Check sheet for the drawn part. Datum: minimum x, y, z corner. Units: mm. A direction names the side the tool comes from. Round coordinates to 2 decimals unless told otherwise and drop trailing zeros. Write each loop counter-clockwise with the first axis right and the second up, starting at its lowest first coordinate (ties: lowest second). Pieces come first, ordered by that corner, then holes.
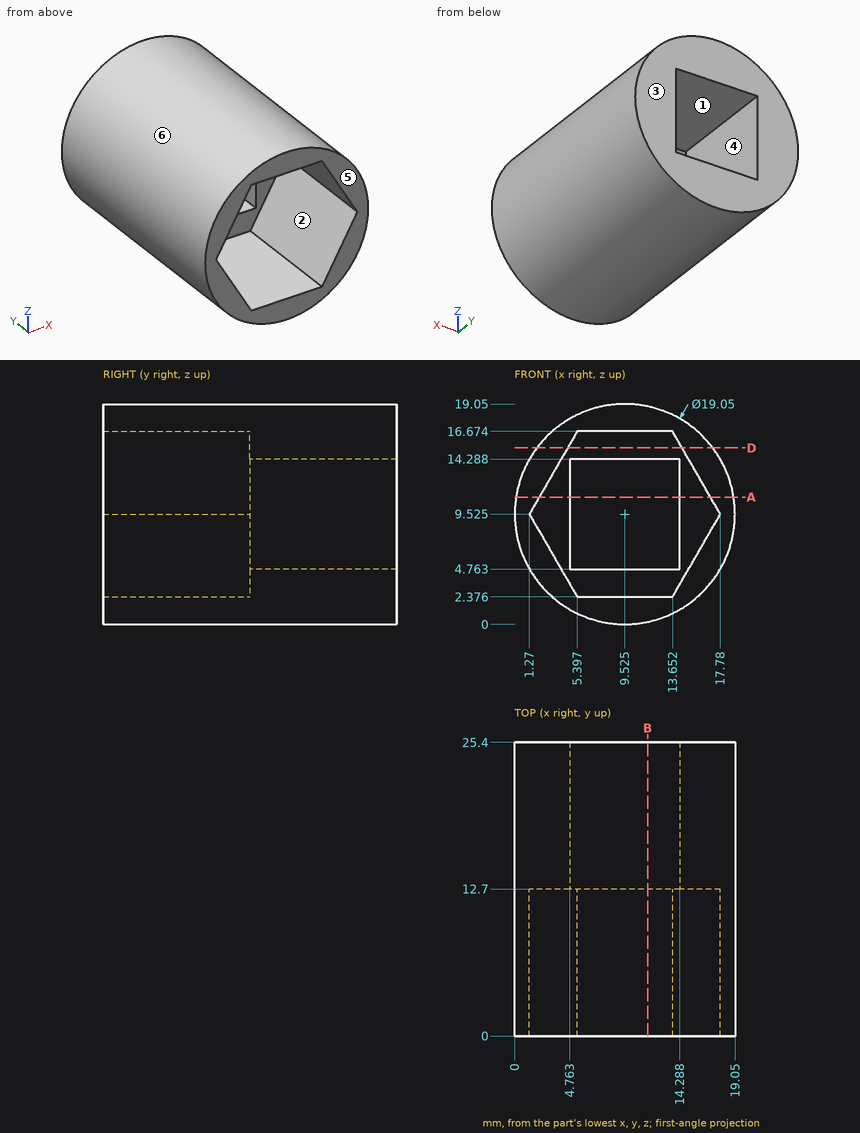
1. Sectioned sample at B-B, the plane x = 11.5. Enter the section's corners in (y, z) (1 decimal), plus the area to 3 significant figures.
2. Sectioned sample at D-D, the plane z = 15.25. Enter the section's corners in (x, y) (1 decimal).
3. Release check for a two-part mould opening along Z. For the marked faces 4, 5 and 6 record: released by +Z, released by -Z, zero draft, split by the parting line, or undercut.
4. Scan lines: line 1 along X through (y, z) = (16.75, 11) (1 decimal); line 2 along X through (y, z) = (1.5, 5) (1 decimal); line 3 along Z through (x, y) = (6, 13) (1 decimal). Record each from-to range of solid material in increasing order.
5. Sectioned sample at A-A, the plane z = 11. Enter the section's corners in (x, y) (1 decimal).
6. Set-up check for the marked faces 1, 2 and 3: record each of +Z, -Z, +X, -X, +Y, -Y from which the full face is reachable in a straight line by a thin tool's end or side.
7. Go/stop test with flat-tipped pins: pin 1 (2.5 mm diameter, centred on x = 9, y = 8, fed in from +Z); pin 2 (3 mm diameter, centred on x = 4.5, y = 19.5, fed in from +Z); pin 3 (3 mm diameter, centred on y = 17.5, z = 11.5, fed in from -X); pin 4 (4 mm diameter, centred on x = 16, y = 10, fed in from -Z). Record where each tip stops, or that it passes through.
Computed values:
1. outline: (0, 0.2) - (25.4, 0.2) - (25.4, 4.8) - (12.7, 4.8) - (12.7, 2.4) - (0, 2.4) - close; (0, 16.7) - (12.7, 16.7) - (12.7, 14.3) - (25.4, 14.3) - (25.4, 18.8) - (0, 18.8) - close
1. area: 171 mm2
2. outline: (1.9, 0) - (4.6, 0) - (4.6, 12.7) - (14.5, 12.7) - (14.5, 0) - (17.1, 0) - (17.1, 25.4) - (1.9, 25.4) - close
3. face 4: undercut
3. face 5: zero draft
3. face 6: split by the parting line
4. line 1: x = 0.1 to 4.8, 14.3 to 18.9
4. line 2: x = 1.1 to 3.9, 15.2 to 17.9
4. line 3: z = 0.7 to 4.8, 14.3 to 18.4
5. outline: (0.1, 0) - (2.1, 0) - (2.1, 12.7) - (4.8, 12.7) - (4.8, 25.4) - (0.1, 25.4) - close; (14.3, 12.7) - (16.9, 12.7) - (16.9, 0) - (18.9, 0) - (18.9, 25.4) - (14.3, 25.4) - close
6. face 1: +Y, -Y
6. face 2: -Y
6. face 3: +Z, -Z, +X, -X, +Y
7. pin 1: stops at z = 19.05
7. pin 2: stops at z = 18.37
7. pin 3: stops at x = 0.01
7. pin 4: stops at z = 1.12
